Read the model definition and answer for the solid it produces. Units are mm, in the model's axes. A direction names the side the tool comes from. Give positions to 0.01 mm unless a question says otherwise; leave off trailing zeros. Order: outer loops, then holes, each group sorted by start corner. A loop starts at its lowest first (then second) coordinate and runs counter-clockwise, first axis right, second up. Notation, with made-up numbers: (-7.75, 2.5) - (-2.75, 2.5) arc R20 ccw to (-2.75, 32.5) - close; hole circle Ø8 at (25, 80.25). An arc over 180 degrees is marked (long way). One line per item, written item: value. Start each with the question number.
```python
from build123d import *

# Parameters (mm, degrees)
BOSS_EXTRUDE2_DEPTH = 40
FILLET1_R           = 4
SKETCH3_W           = 50
SKETCH3_H           = 8
BOSS_EXTRUDE3_DEPTH = 80
SKETCH5_R           = 5.25
CUT_EXTRUDE1_DEPTH  = 127.113847389
FILLET2_R           = 10
FILLET3_R           = 3


with BuildPart() as part:
    # Sketch2 → Boss-Extrude2 (new, symmetric)
    with BuildSketch(Plane.XY):
        with BuildLine():
            Line((-32, 0), (32, 0))
            Line((32, 0), (62, 51.961524227))
            ThreePointArc((62, 51.961524227), (64.732050808, 52.693575035), (65.464101615, 49.961524227))
            Line((65.464101615, 49.961524227), (34.309401077, -4))
            Line((34.309401077, -4), (-34.309401077, -4))
            Line((-34.309401077, -4), (-65.464101615, 49.961524227))
            ThreePointArc((-65.464101615, 49.961524227), (-64.732050808, 52.693575035), (-62, 51.961524227))
            Line((-62, 51.961524227), (-32, 0))
        make_face()
    extrude(amount=BOSS_EXTRUDE2_DEPTH, both=True)

    # Fillet1
    fillet1_edges = [part.edges().sort_by_distance(p)[0] for p in [
        (-32, 0, 0),
        (32, 0, 0),
    ]]
    fillet(fillet1_edges, radius=FILLET1_R)

    # Sketch3 → Boss-Extrude3 (add)
    with BuildSketch(Plane(origin=(0, 0, 0), x_dir=(1, 0, 0), z_dir=(0, 1, 0))):
        with Locations((0, 36)):
            Rectangle(SKETCH3_W, SKETCH3_H)
    extrude(amount=BOSS_EXTRUDE3_DEPTH)

    # Sketch5 → Cut-Extrude1 (cut, through all)
    with BuildSketch(Plane.XY.offset(-32)):
        with Locations((-9.5, 70)):
            Circle(SKETCH5_R)
        with Locations((9.5, 70)):
            Circle(SKETCH5_R)
    extrude(amount=-CUT_EXTRUDE1_DEPTH, mode=Mode.SUBTRACT)

    # Fillet2
    # the kernel refuses this fillet: 10 mm, written as the material it adds along each edge
    with BuildSketch(Plane(origin=(25, 0, -40), x_dir=(1, 0, 0), z_dir=(0, 0, 1)), Plane(origin=(-25, 0, -32), x_dir=(-1, 0, 0), z_dir=(0, 0, -1))) as fillet2_piece_1:
        with BuildLine():
            CenterArc((10, 8.474093474), FILLET2_R, 180, 57.931003855)
            Line((0, 8.474093474), (0, 0))
            Line((0, 0), (4.690598923, 0))
        make_face()
    extrude(amount=8)
    # the kernel refuses this fillet: 10 mm, written as the material it takes off along each edge
    with BuildSketch(Plane(origin=(25, 80, -65), x_dir=(0, -1, 0), z_dir=(0, 0, 1))) as fillet2_2_piece_1:
        with BuildLine():
            CenterArc((FILLET2_R, -FILLET2_R), FILLET2_R, 90, 90)
            Line((0, -FILLET2_R), (0, 0))
            Line((0, 0), (FILLET2_R, 0))
        make_face()
    extrude(amount=58, mode=Mode.SUBTRACT)
    with BuildSketch(Plane(origin=(-25, 80, -7), x_dir=(1, 0, 0), z_dir=(0, 0, -1))) as fillet2_2_piece_2:
        with BuildLine():
            CenterArc((FILLET2_R, FILLET2_R), FILLET2_R, 180, 90)
            Line((0, FILLET2_R), (0, 0))
            Line((0, 0), (FILLET2_R, 0))
        make_face()
    extrude(amount=58, mode=Mode.SUBTRACT)

    # Fillet3
    # the kernel refuses this fillet: 3 mm, written as the material it adds along each edge
    with BuildSketch(Plane(origin=(-37.190598923, 0, -32), x_dir=(0, 1, 0), z_dir=(1, 0, 0))) as fillet3_piece_1_section:
        with BuildLine():
            CenterArc((FILLET3_R, FILLET3_R), FILLET3_R, 180, 90)
            Line((0, FILLET3_R), (0, 0))
            Line((0, 0), (FILLET3_R, 0))
        make_face()
    fillet3_piece_1 = extrude(amount=74.381197846, mode=Mode.PRIVATE)
    fillet3_piece_1 = fillet3_piece_1 - Plane(origin=(35, 8.474093474, -32), x_dir=(1, 0, 0), z_dir=(0, 0, -1)) * Cylinder(10, 161, mode=Mode.PRIVATE)
    fillet3_piece_1 = fillet3_piece_1 - Plane(origin=(-35, 8.474093474, -32), x_dir=(-1, 0, 0), z_dir=(0, 0, 1)) * Cylinder(10, 161, mode=Mode.PRIVATE)
    add(fillet3_piece_1)


solid = part.part
```
1) Section B-B on z = 29 is taken. Write down the section's boundary in (x, y).
2) The mould has two halves that part along X. Classify faces 4 (the cylindrical face through (22.15, 76.99, -36.06)), 5 (the flat face through (0, 80, -36)), 6 (the flat face through (-49.669, 22.603, 0.56)), 7 (the flat face through (0, 42, -32)): +X half, -X half, draft (parallel to the pull), parting line (faces both ways), or undercut.
3) Section D-D on y = 60 is taken. Write down the section's boundary in (x, z).
4) Section A-A on x = 9.5 is taken. Write down the section's boundary in (y, z), plus the area to 3 significant figures.
5) Section C-C on y = 10.5 is taken. Write down the section's boundary in (x, z), plus the area to 3 significant figures.
6) Each of these flat-tipped pins is pushed along its axis until it touches: pin 1 (9 mm diameter, centred on y = 44, z = -34.5, fed in from -X); pin 2 (6 mm diameter, centred on y = 22, z = -22, fed in from +X); pin 3 (17 mm diameter, centred on x = -9.5, y = 70, fed in from +Z); pin 4 (8.5 mm diameter, centred on x = 9.5, y = 70, fed in from -Z). Where does it stop, or does it pass through?
7) Find the intervals of material crossed by probe 1 along Y at (x, z) = (9.5, -34); probe 2 along X at (y, z) = (48, -33); probe 3 along Y at (x, z) = (16, 5.5), in increasing order. Write a range as from..to.
8) For faces 1 (the cylindrical face through (-0.42, 0.86, -31.1)), 2 (the cylindrical face through (26.285, 3.569, -35.799)), 3 (the cylindrical face through (8.362, 64.875, -35.944)), determine the directions among +Z, -Z, +X, -X, +Y, -Y from which every point of the face is accessible in a straight line to the end or side of a thin tool.
Solved:
1. outline: (-65.46, 49.96) - (-34.31, -4) - (34.31, -4) - (65.46, 49.96) arc R2 ccw to (62, 51.96) - (33.15, 2) arc R4 cw to (29.69, 0) - (-29.69, 0) arc R4 cw to (-33.15, 2) - (-62, 51.96) arc R2 ccw to start
2. face 4: +X half
2. face 5: draft
2. face 6: -X half
2. face 7: undercut
3. outline: (-25, -40) - (25, -40) - (25, -32) - (-25, -32) - close
4. outline: (-4, -40) - (64.75, -40) - (64.75, -32) - (3, -32) arc R3 cw to (0, -29) - (0, 40) - (-4, 40) - close; (75.25, -40) - (80, -40) - (80, -32) - (75.25, -32) - close
4. area: 878 mm2
5. outline: (-42.68, -40) - (-38.06, -40) - (-38.06, 40) - (-42.68, 40) - close; (-25, -40) - (25, -40) - (25, -32) - (-25, -32) - close; (38.06, -40) - (42.68, -40) - (42.68, 40) - (38.06, 40) - close
5. area: 1,140 mm2
6. pin 1: stops at x = -64.62
6. pin 2: stops at x = 51.05
6. pin 3: stops at z = -32
6. pin 4: passes through
7. probe 1: y = -4..64.75, 75.25..80
7. probe 2: x = -64.33..-59.71, -25..25, 59.71..64.33
7. probe 3: y = -4..0
8. face 1: +Z, +Y
8. face 2: +Z, -Z, +Y
8. face 3: +Z, -Z
